Study the drawing (mm; zero at the part's minimum x, y, z) and answer. Give positions to 0.01 mm unless a question says otherwise; leave off trailing zeros. Loops run counter-clockwise (first coordinate to the right, second up) from the corner with the lowest first, then second, coordinate; pieces in that order, holes last. Notation, with made-up numbers: M 52,-23 L 61,-23 A15 ccw 61,-1 Z; hole C 26.5,-15.75 d2. An arc over 180 degrees is marked long. Use one line per item in the form item = value. Start each with the question number.
1. The part is cut by section C-C (z = 16.5). Write down the section's boundary in (x, y) (1 decimal).
2. Straight lines are drawn through the part: line 1 (Z direction, x = 43, y = 0.4); line 2 (X direction, y = 0.5, z = 4.25) (1 decimal); line 3 (Z direction, x = 63, y = 1.95) (1 decimal). For each, find the intervals that lie inside material, in ascending order. Write a range as from..to.
3. The part is cut by section A-A (y = 1.95). Write down the section's boundary in (x, z).
4. The part is cut by section B-B (x = 40.5). Write down the section's boundary in (y, z), and give its area (3 significant figures).
5. Each of these flat-tipped pins is pushed along its axis until it touches: pin 1 Ø0.9 at (x, y) = (49, 1) entering from -Z; pin 2 Ø1.5 at (x, y) = (30, 1) entering from -Z; pin 3 Ø1.5 at (x, y) = (44, 1.5) entering from +Z. Where does it stop, or does it pass through?
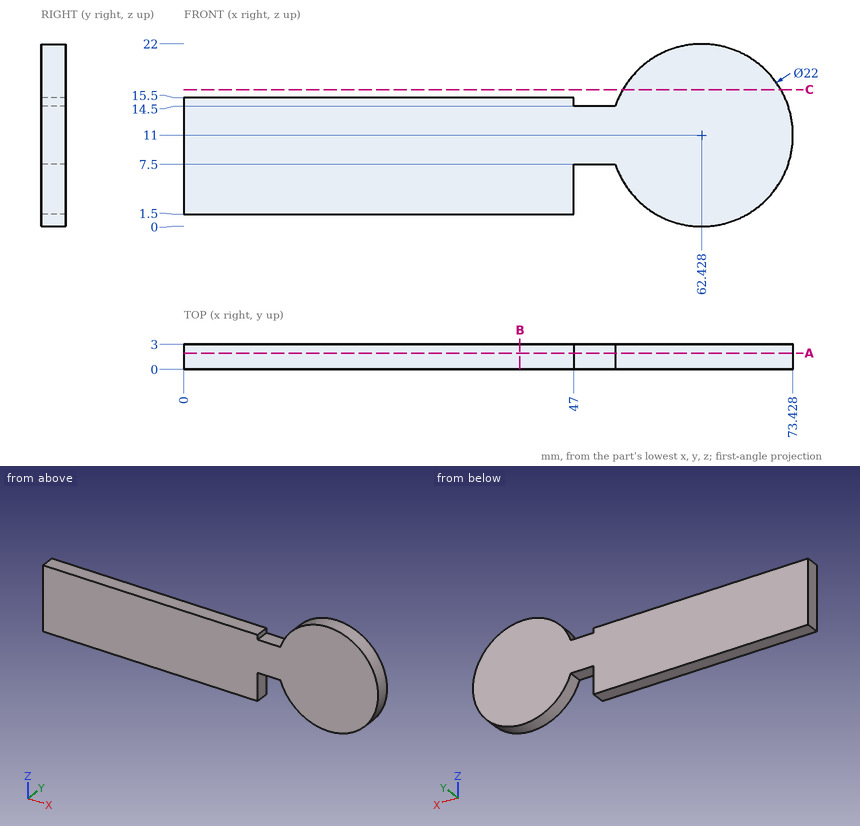
Derived:
q1.outline = M 52.9,0 L 72,0 L 72,3 L 52.9,3 Z
q2.line_1 = 1.5..15.5
q2.line_2 = 0..47, 53.7..71.1
q2.line_3 = 0..22
q3.outline = M 0,1.5 L 47,1.5 L 47,7.5 L 52,7.5 A11 ccw long 52,14.5 L 47,14.5 L 47,15.5 L 0,15.5 Z
q4.outline = M 0,1.5 L 3,1.5 L 3,15.5 L 0,15.5 Z
q4.area = 42.0 mm2
q5.pin_1 = 7.5
q5.pin_2 = 1.5
q5.pin_3 = 15.5
